The listing builds one solid part. Answer for the finished solid, in the listing's coordinates (mm). A direction names the side the tool comes from. Give positions to 0.01 mm unless a question says otherwise; leave off trailing zeros. Write each loop counter-clockwise with the first axis right and the second up, starting at its lowest first coordinate (ties: lowest second). Pieces come first, ordered by that corner, then holes. Notation, with made-up numbers: (82, 37) - (90, 37) arc R4 ccw to (90, 41) - close; hole circle Ø9 at (3, -15). An arc over 180 degrees is marked (long way). Use a Markdown table: item, result. Add a question column.
Autodesk Inventor part; units mm, degrees
ref_plane "Work Plane1" through (8.5, -35.5, -35.5) normal (0, 0, -1) x (-1, 0, 0)
ref_plane "YZ Plane" through (0, 0, 0) normal (1, 0, 0) x (0, 1, 0)
ref_plane "XZ Plane" through (0, 0, 0) normal (0, 1, 0) x (-1, 0, 0)
ref_plane "Work Plane1" through (8.5, -35.5, -35.5) normal (0, 0, -1) x (-1, 0, 0)
sketch "Sketch1" plane through (8.5, -35.5, -35.5) normal (0, 0, -1) x (-1, 0, 0)
  circle A0 centre (0, 0) radius 3
  circle A1 centre (0, 0) radius 6
  circle A2 centre (-36.75, -21.2176) radius 3
  circle A3 centre (-36.75, -21.2176) radius 6
  circle A4 centre (-36.75, 21.2176) radius 6
  circle A5 centre (-36.75, 21.2176) radius 3
  line L0 (-36.75, -46.2176) -> (28, -46.2176)
  line L1 (28, -46.2176) -> (28, 0)
  line L2 (-36.75, -46.2176) -> (-59, -46.2176)
  line L3 (-59, -46.2176) -> (-59, 34.5)
  line L4 (-59, 34.5) -> (28, 34.5)
  line L5 (34.5, 35.5) -> (-17.5, 35.5)
  line L6 (28, 34.5) -> (28, 0)
  circle A6 centre (-24.5, 0) radius 11
  circle A7 centre (-24.5, 0) radius 15
  point P0 (8.5, 35.5)
  dimension "d3" = 30
extrude "Extrusion1" add sketch "Sketch1" along normal blind 5 contours A1 | A3 | A4 | L2 L3 L4 L6 L1 L0
sketch "Sketch2" plane through (-19.5, -81.7176, -35.5) normal (-1, 0, 0) x (0, 0, 1)
  line L0 (0, 0) -> (0, 80.7176)
  line L1 (0, 80.7176) -> (-5, 80.7176)
  line L2 (-5, 0) -> (-5, 80.7176)
  line L3 (0, 0) -> (-5, 0)
  point P0 (35.5, 81.7176)
extrude "Extrusion2" add sketch "Sketch2" along normal blind 5
sketch "Sketch3" plane through (67.5, -81.7176, -40.5) normal (0, -1, 0) x (1, 0, 0)
  line L0 (0, 5) -> (-92, 5)
  line L1 (-92, 0) -> (-92, 5)
  line L2 (0, 0) -> (-92, 0)
  line L3 (0, 5) -> (0, 0)
  point P0 (-67.5, 40.5)
extrude "Extrusion3" add sketch "Sketch3" along normal blind 5
sketch "Sketch4" plane through (8.5, -35.5, -35.5) normal (0, 0, 1) x (1, 0, 0)
  line L0 (-28, -46.2176) -> (-28, 34.5)
  line L1 (-28, -46.2176) -> (59, -46.2176)
  line L2 (59, -51.2176) -> (-33, -51.2176)
  line L3 (-33, 34.5) -> (-33, -51.2176)
  line L4 (59, 34.5) -> (59, -51.2176)
  line L5 (59, 34.5) -> (-33, 34.5)
  line L6 (-28, -46.2176) -> (-33, -46.2176)
  line L7 (-33, 34.5) -> (-33, -51.2176)
extrude "Extrusion4" add sketch "Sketch4" along normal blind 75 contours L1 L4 L2 L3 L6
sketch "Sketch5" plane through (67.5, -86.7176, -40.5) normal (0, -1, 0) x (1, 0, 0)
  line L0 (-92, 5) -> (-92, 80)
  line L1 (-92, 80) -> (-77.75, 80)
  line L2 (-92, 80) -> (0, 80)
  line L3 (-77.75, 80) -> (-37.75, 80)
  line L4 (-37.75, 80) -> (-37.75, 65)
  line L5 (-37.75, 65) -> (-77.75, 65)
  circle A0 centre (-77.75, 65) radius 4.25
  circle A1 centre (-37.75, 65) radius 4.25
  point P0 (-67.5, 40.5)
  dimension "d14" = 14.25
  dimension "d15" = 40
  dimension "d16" = 15
  dimension "d17" = 8.5
  dimension "d18" = 8.5
extrude "Extrusion5" cut sketch "Sketch5" against normal through all
sketch "Sketch6" plane through (67.5, -1, -35.5) normal (0, 1, 0) x (1, 0, 0)
  line L0 (0, 0) -> (-92, 0)
  line L1 (0, 0) -> (0, 5)
  line L2 (0, 5) -> (-92, 5)
  line L3 (-92, 0) -> (-92, 5)
  point P0 (-67.5, -35.5)
extrude "Extrusion6" add sketch "Sketch6" along normal blind 20
sketch "Sketch7" plane through (67.5, 19, -35.5) normal (0, 1, 0) x (1, 0, 0)
  circle A0 centre (-67.5, -35.5) radius 31
  circle A1 centre (-67.5, -35.5) radius 31
  circle A2 centre (-67.5, -35.5) radius 31
  line L0 (-67.5, -66.5) -> (-67.5, -75)
  line L1 (0, -75) -> (-92, -75)
  line L2 (0, 5) -> (0, -75)
  line L3 (-67.5, -75) -> (0, -75)
  line L4 (0, -75) -> (0, 5)
  line L5 (-65, -20.5) -> (-65, 0)
  line L6 (-65, -4.601) -> (-65, 0)
  line L7 (-92, 5) -> (-92, 0)
  line L8 (-92, 0) -> (0, 0)
  line L9 (0, 0) -> (0, 5)
  line L10 (0, 5) -> (-92, 5)
  point P0 (-65, -4.601)
extrude "Extrusion7" add sketch "Sketch7" along normal blind 20 contours A0 L5 L8 L2 L1 L0 | L8 L7 L10 L2
sketch "Sketch10" plane through (8.5, -35.5, 39.5) normal (0, 0, 1) x (1, 0, 0)
  line L0 (59, -51.2176) -> (59, -46.2176)
  line L1 (59, -46.2176) -> (-33, -46.2176)
  line L2 (-33, -46.2176) -> (-33, -51.2176)
  line L3 (-33, -51.2176) -> (59, -51.2176)
  point P0 (-8.5, 35.5)
extrude "Extrusion10" cut sketch "Sketch10" against normal up to surface (75 mm away)
sketch "Sketch11" plane through (0, 19, 39.5) normal (0, 0, 1) x (1, 0, 0)
  line L0 (0, 0) -> (67.5, 0)
  line L1 (67.5, 0) -> (67.5, 20)
  line L2 (0, 20) -> (67.5, 20)
  line L3 (0, 0) -> (0, 20)
  point P0 (0, -19)
extrude "Extrusion11" add sketch "Sketch11" along normal blind 10
sketch "Sketch12" plane through (67.5, 19, -35.5) normal (0, -1, 0) x (1, 0, 0)
  line L0 (-67.5, 66.5) -> (-67.5, 85)
  line L1 (-67.5, 85) -> (0, 85)
  line L2 (-67.5, 85) -> (0, 85)
  line L3 (0, 85) -> (0, 75)
  line L4 (0, 0) -> (0, 85)
  line L5 (0, 75) -> (-67.5, 75)
  line L6 (-67.5, 75) -> (-67.5, 85)
  point P0 (-67.5, 35.5)
  dimension "d35" = 10
extrude "Extrusion12" add sketch "Sketch12" along normal blind 20
sketch "Sketch13" plane through (0, 19, 49.5) normal (0, 0, 1) x (1, 0, 0)
  line L0 (67.5, 20) -> (67.5, -20)
  line L1 (67.5, 20) -> (0, 20)
  line L2 (0, 20) -> (0, -20)
  line L3 (67.5, -20) -> (0, -20)
  point P0 (0, -19)
extrude "Extrusion13" add sketch "Sketch13" along normal blind 59.488
sketch "Sketch14" plane through (67.5, -1, -35.5) normal (0, -1, 0) x (1, 0, 0)
  line L0 (-53.25, 129.488) -> (-13.25, 129.488)
  circle A0 centre (-53.25, 129.488) radius 4.25
  circle A1 centre (-13.25, 129.488) radius 4.25
  point P0 (-67.5, 35.5)
  point P1 (-67.5, 144.488)
  dimension "d43" = 40
  dimension "d44" = 8.5
  dimension "d45" = 8.5
extrude "Extrusion14" cut sketch "Sketch14" against normal up to surface (40 mm away)
sketch "Sketch15" plane through (67.5, -86.7176, -40.5) normal (1, 0, 0) x (0, 0, -1)
  line L0 (-5, 105.7176) -> (-5, 0)
  line L1 (0, 0) -> (-5, 0)
  line L2 (0, 0) -> (0, 125.7176)
  line L3 (0, 125.7176) -> (-149.488, 125.7176)
  line L4 (-149.488, 85.7176) -> (-149.488, 125.7176)
  line L5 (-80, 85.7176) -> (-149.488, 85.7176)
  line L6 (-80, 105.7176) -> (-80, 85.7176)
  line L7 (-5, 105.7176) -> (-80, 105.7176)
  point P0 (-40.5, 86.7176)
extrude "Extrusion15" add sketch "Sketch15" along normal blind 1
sketch "Sketch16" plane through (0, 19, 31) normal (-1, 0, 0) x (0, 0, 1)
  line L0 (77.988, 20) -> (77.988, -20)
  line L1 (77.988, 0) -> (42.988, 0)
  circle A0 centre (42.988, 0) radius 4.25
  point P0 (-31, -19)
  dimension "d50" = 35
  dimension "d51" = 8.5
extrude "Extrusion16" cut sketch "Sketch16" against normal up to surface (68.5 mm away)
sketch "Sketch17" plane through (67.5, 39, -35.5) normal (0, 1, 0) x (1, 0, 0)
  circle A0 centre (-53.25, -129.488) radius 4.25
  line L0 (-53.25, -129.488) -> (-33.25, -129.488)
  line L1 (-33.25, -129.488) -> (-33.25, -99.488)
  circle A1 centre (-33.25, -99.488) radius 4.25
  point P0 (-67.5, -35.5)
  dimension "d54" = 20
  dimension "d55" = 30
  dimension "d56" = 8.5
extrude "Extrusion17" cut sketch "Sketch17" against normal up to surface (40 mm away) contours A1
properties part number "motor_connector_left"
1. Given P1, Ø5, axis at y = 19, z = 73.988, coming from the +X side (1 decimal); P2, Ø2.5, axis at y = 29, z = -33.5, coming from the -X side; P3, Ø10, axis at x = 34.25, z = 63.988, coming from the +Y side; P4, Ø20.5, axis at x = 25.5, z = 57.5, coming from the -Y side, each flat-ended and moving along its own axis, determine where each tip first touches the part or whether it passes through.
2. Which of the six approach directions +Z, -Z, +X, -X, +Y, -Y give full straight-line access (tool end or side, diameter ignored) to faces 1 (the flat face through (0, 19, 69)), 2 (the flat face through (2.5, 29, -33)), 3 (the flat face through (41, 19, 1)), 4 (the flat face through (34, -1, 74))?
3. The part is cut by section B-B (x = 36.5). Give the vertices of the cut face in (y, z).
4. The part is cut by section D-D (x = 14). Give the vertices of the cut face in (y, z).
5. The part is cut by section C-C (y = 27). Give the vertices of the cut face in (x, z).
6. For a pull along Z with two mould halves and no side action, classify faces 5 (the flat face through (34, 19, 108.988)), 6 (the cylindrical face through (48.247, -14.414, -37.965)), 7 (the cylindrical face through (33.77, 19.187, 69.742)), 8 (the flat face through (21, -25, -40.5)) as released by +Z, released by -Z, zero draft, split by the parting line, or undercut.
7. Consider L1, parallel to Z at x = 34.5, y = 6; L2, parallel to Y at x = 45.25, z = -36.6; L3, parallel to Z at x = 58, y = -48. Determine where each line is inside the solid, lowest interval first. Write a range as [from, to].
8. The part is cut by section A-A (x = 52.5). Give the vertices of the cut face in (y, z).
Check values:
| question | item | result |
|---|---|---|
| 1 | P1 | passes through |
| 1 | P2 | stops at x = 2.5 |
| 1 | P3 | stops at y = 39 |
| 1 | P4 | stops at y = -1 |
| 2 | face 1 | +Z, -X, +Y, -Y |
| 2 | face 2 | -X, +Y, -Y |
| 2 | face 3 | +X, -X, -Y |
| 2 | face 4 | +Z, +X, -X, -Y |
| 3 | outline | (-86.72, -40.5) - (-50.09, -40.5) - (-50.09, -35.5) - (-86.72, -35.5) - close; (-20.91, -40.5) - (39, -40.5) - (39, 60.38) - (-1, 60.38) - (-1, 39.5) - (19, 39.5) - (19, -35.5) - (-20.91, -35.5) - close; (-1, 67.59) - (39, 67.59) - (39, 108.99) - (-1, 108.99) - close; hole circle Ø8.5 at (19, 73.99) |
| 4 | outline | (-86.72, -40.5) - (39, -40.5) - (39, -27.66) - (19, -27.66) - (19, -35.5) - (-86.72, -35.5) - close; (-1, 39.5) - (19, 39.5) - (19, 27.66) - (39, 27.66) - (39, 89.75) - (-1, 89.75) - close; (-1, 98.23) - (39, 98.23) - (39, 108.99) - (-1, 108.99) - close; hole circle Ø8.5 at (19, 73.99) |
| 5 | outline | (-24.5, -40.5) - (68.5, -40.5) - (68.5, 108.99) - (0, 108.99) - (0, 31) arc R31 cw to (2.5, -30.9) - (2.5, -35.5) - (-24.5, -35.5) - close; hole circle Ø8.5 at (14.25, 93.99); hole circle Ø8.5 at (34.25, 63.99); hole circle Ø8.5 at (54.25, 93.99) |
| 6 | face 5 | released by +Z |
| 6 | face 6 | zero draft |
| 6 | face 7 | undercut |
| 6 | face 8 | released by -Z |
| 7 | L1 | z = [-40.5, -35.5], [39.5, 59.75], [68.23, 108.99] |
| 7 | L2 | y = [-86.72, -59.72], [-53.72, -44.16], [-26.84, -17.28], [-11.28, 39] |
| 7 | L3 | z = [-40.5, -35.5] |
| 8 | outline | (-86.72, -40.5) - (39, -40.5) - (39, 90.12) - (-1, 90.12) - (-1, 39.5) - (19, 39.5) - (19, -35.5) - (-86.72, -35.5) - close; (-1, 97.86) - (39, 97.86) - (39, 108.99) - (-1, 108.99) - close; hole circle Ø8.5 at (19, 73.99) |
